Could you check a few things on this model? Use its own coordinates, in mm. Give positions to 0.01 mm unless a question says otherwise; leave off trailing zeros. Order: outer loops, then holes, each group sorted by start corner. A loop starts at its lowest first (then second) coordinate and runs counter-clockwise, first axis right, second up. Notation, with made-up numbers: M 72,18 L 94,18 A12 ccw 94,39 Z; hole C 10,65.5 d4. An arc over 180 degrees is marked long. Answer in a Markdown table with one row per item. Add a question column.
```python
from build123d import *

# Parameters (mm, degrees)
SKETCH1_W           = 203.2
SKETCH1_H           = 133.35
BOSS_EXTRUDE1_DEPTH = 3.175
SKETCH2_R           = 2.54
CUT_EXTRUDE1_DEPTH  = 122.565604716
SKETCH3_W           = 35.687
SKETCH3_H           = 3.175
BOSS_EXTRUDE2_DEPTH = 3.175
SKETCH4_W           = 3.175
SKETCH4_H           = 18.542
BOSS_EXTRUDE3_DEPTH = 3.175
BOSS_EXTRUDE4_DEPTH = 3.175
SKETCH6_W           = 76.708
SKETCH6_H           = 51.308
CUT_EXTRUDE2_DEPTH  = 126.963898598


with BuildPart() as part:
    # Sketch1 → Boss-Extrude1 (new body)
    with BuildSketch(Plane(origin=(0, 0, 0), x_dir=(1, 0, 0), z_dir=(0, 1, 0))):
        Rectangle(SKETCH1_W, SKETCH1_H)
    extrude(amount=BOSS_EXTRUDE1_DEPTH)

    # Sketch2 → Cut-Extrude1 (cut, through all)
    with BuildSketch(Plane(origin=(0, 3.175, 0), x_dir=(1, 0, 0), z_dir=(0, 1, 0))):
        with Locations(Location((-88.9, 50.8, 0), (0, 0, 270))):
            Circle(SKETCH2_R)
        with Locations(Location((-76.2, 50.8, 0), (0, 0, 270))):
            Circle(SKETCH2_R)
        with Locations(Location((-63.5, 50.8, 0), (0, 0, 270))):
            Circle(SKETCH2_R)
        with Locations(Location((-50.8, 50.8, 0), (0, 0, 270))):
            Circle(SKETCH2_R)
        with Locations(Location((-76.2, 38.1, 0), (0, 0, 270))):
            Circle(SKETCH2_R)
        with Locations(Location((-63.5, 38.1, 0), (0, 0, 270))):
            Circle(SKETCH2_R)
        with Locations(Location((-50.8, 38.1, 0), (0, 0, 270))):
            Circle(SKETCH2_R)
        with Locations(Location((-76.2, 25.4, 0), (0, 0, 270))):
            Circle(SKETCH2_R)
        with Locations(Location((-63.5, 25.4, 0), (0, 0, 270))):
            Circle(SKETCH2_R)
        with Locations(Location((-50.8, 25.4, 0), (0, 0, 270))):
            Circle(SKETCH2_R)
        with Locations(Location((-76.2, 12.7, 0), (0, 0, 270))):
            Circle(SKETCH2_R)
        with Locations(Location((-63.5, 12.7, 0), (0, 0, 270))):
            Circle(SKETCH2_R)
        with Locations(Location((-50.8, 12.7, 0), (0, 0, 270))):
            Circle(SKETCH2_R)
        with Locations(Location((-76.2, 0, 0), (0, 0, 270))):
            Circle(SKETCH2_R)
        with Locations(Location((-63.5, 0, 0), (0, 0, 270))):
            Circle(SKETCH2_R)
        with Locations(Location((-50.8, 0, 0), (0, 0, 270))):
            Circle(SKETCH2_R)
        with Locations(Location((-76.2, -12.7, 0), (0, 0, 270))):
            Circle(SKETCH2_R)
        with Locations(Location((-63.5, -12.7, 0), (0, 0, 270))):
            Circle(SKETCH2_R)
        with Locations(Location((-50.8, -12.7, 0), (0, 0, 270))):
            Circle(SKETCH2_R)
        with Locations(Location((-76.2, -25.4, 0), (0, 0, 270))):
            Circle(SKETCH2_R)
        with Locations(Location((-63.5, -25.4, 0), (0, 0, 270))):
            Circle(SKETCH2_R)
        with Locations(Location((-50.8, -25.4, 0), (0, 0, 270))):
            Circle(SKETCH2_R)
        with Locations(Location((-76.2, -38.1, 0), (0, 0, 270))):
            Circle(SKETCH2_R)
        with Locations(Location((-63.5, -38.1, 0), (0, 0, 270))):
            Circle(SKETCH2_R)
        with Locations(Location((-50.8, -38.1, 0), (0, 0, 270))):
            Circle(SKETCH2_R)
        with Locations(Location((-76.2, -50.8, 0), (0, 0, 270))):
            Circle(SKETCH2_R)
        with Locations(Location((-63.5, -50.8, 0), (0, 0, 270))):
            Circle(SKETCH2_R)
        with Locations(Location((-50.8, -50.8, 0), (0, 0, 270))):
            Circle(SKETCH2_R)
        with Locations(Location((-88.9, 38.1, 0), (0, 0, 270))):
            Circle(SKETCH2_R)
        with Locations(Location((-88.9, 25.4, 0), (0, 0, 270))):
            Circle(SKETCH2_R)
        with Locations(Location((-88.9, 12.7, 0), (0, 0, 270))):
            Circle(SKETCH2_R)
        with Locations(Location((-88.9, 0, 0), (0, 0, 270))):
            Circle(SKETCH2_R)
        with Locations(Location((-88.9, -12.7, 0), (0, 0, 270))):
            Circle(SKETCH2_R)
        with Locations(Location((-88.9, -25.4, 0), (0, 0, 270))):
            Circle(SKETCH2_R)
        with Locations(Location((-88.9, -38.1, 0), (0, 0, 270))):
            Circle(SKETCH2_R)
        with Locations(Location((-88.9, -50.8, 0), (0, 0, 270))):
            Circle(SKETCH2_R)
        with Locations(Location((-38.1, 50.8, 0), (0, 0, 270))):
            Circle(SKETCH2_R)
        with Locations(Location((-38.1, 38.1, 0), (0, 0, 270))):
            Circle(SKETCH2_R)
        with Locations(Location((-38.1, 25.4, 0), (0, 0, 270))):
            Circle(SKETCH2_R)
        with Locations(Location((-38.1, 12.7, 0), (0, 0, 270))):
            Circle(SKETCH2_R)
        with Locations(Location((-38.1, 0, 0), (0, 0, 270))):
            Circle(SKETCH2_R)
        with Locations(Location((-38.1, -12.7, 0), (0, 0, 270))):
            Circle(SKETCH2_R)
        with Locations(Location((-38.1, -25.4, 0), (0, 0, 270))):
            Circle(SKETCH2_R)
        with Locations(Location((-38.1, -38.1, 0), (0, 0, 270))):
            Circle(SKETCH2_R)
        with Locations(Location((-38.1, -50.8, 0), (0, 0, 270))):
            Circle(SKETCH2_R)
    extrude(amount=-CUT_EXTRUDE1_DEPTH, mode=Mode.SUBTRACT)

    # Sketch3 → Boss-Extrude2 (add)
    with BuildSketch(Plane(origin=(0, 3.175, 0), x_dir=(1, 0, 0), z_dir=(0, 1, 0))):
        with Locations((-61.2775, 68.2625)):
            Rectangle(SKETCH3_W, SKETCH3_H)
        with Locations((0.3175, 68.2625)):
            Rectangle(SKETCH3_W, SKETCH3_H)
        with Locations((61.9125, 68.2625)):
            Rectangle(SKETCH3_W, SKETCH3_H)
        with Locations((61.9125, -68.2625)):
            Rectangle(SKETCH3_W, SKETCH3_H)
        with Locations((0.3175, -68.2625)):
            Rectangle(SKETCH3_W, SKETCH3_H)
        with Locations((-61.2775, -68.2625)):
            Rectangle(SKETCH3_W, SKETCH3_H)
    extrude(amount=-BOSS_EXTRUDE2_DEPTH)

    # Sketch4 → Boss-Extrude3 (add)
    with BuildSketch(Plane(origin=(0, 3.175, 0), x_dir=(1, 0, 0), z_dir=(0, 1, 0))):
        with Locations((-103.1875, 38.1)):
            Rectangle(SKETCH4_W, SKETCH4_H)
        with Locations((-103.1875, 0)):
            Rectangle(SKETCH4_W, SKETCH4_H)
        with Locations((-103.1875, -38.1)):
            Rectangle(SKETCH4_W, SKETCH4_H)
        with Locations((103.1875, -38.1)):
            Rectangle(SKETCH4_W, SKETCH4_H)
        with Locations((103.1875, 0)):
            Rectangle(SKETCH4_W, SKETCH4_H)
        with Locations((103.1875, 38.1)):
            Rectangle(SKETCH4_W, SKETCH4_H)
    extrude(amount=-BOSS_EXTRUDE3_DEPTH)

    # Sketch5 → Boss-Extrude4 (add)
    with BuildSketch(Plane(origin=(0, 3.175, 0), x_dir=(1, 0, 0), z_dir=(0, 1, 0))):
        Polygon((-104.775, -47.371), (-104.775, -69.85), (-79.121, -69.85), (-79.121, -66.675), (-101.6, -66.675), (-101.6, -47.371), align=None)
        Polygon((-101.6, 47.371), (-104.775, 47.371), (-104.775, 69.85), (-79.121, 69.85), (-79.121, 66.675), (-101.6, 66.675), align=None)
        Polygon((104.775, 47.371), (104.775, 69.85), (79.121, 69.85), (79.121, 66.675), (101.6, 66.675), (101.6, 47.371), align=None)
        Polygon((101.6, -47.371), (104.775, -47.371), (104.775, -69.85), (79.121, -69.85), (79.121, -66.675), (101.6, -66.675), align=None)
    extrude(amount=-BOSS_EXTRUDE4_DEPTH)

    # Sketch6 → Cut-Extrude2 (cut, through all)
    with BuildSketch(Plane(origin=(0, 3.175, 0), x_dir=(1, 0, 0), z_dir=(0, 1, 0))):
        with Locations((25.4, 0)):
            Rectangle(SKETCH6_W, SKETCH6_H)
    extrude(amount=-CUT_EXTRUDE2_DEPTH, mode=Mode.SUBTRACT)


solid = part.part
```
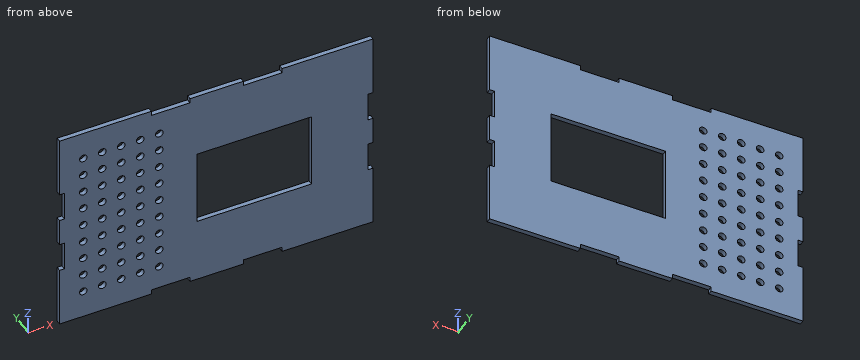
1. If I drill on line 1 along X through (y, z) = (1.45, -50.8) (3 decimals); line 2 along X through (y, z) = (2.65, -37) (3 decimals); line 3 along X through (y, z) = (1.25, 18.5), over which ranges is the centre line in solid material (lowest first)? Write a range as [from, to].
2. Suppose I cut it at B-B on x = 39.5. List the corners of the cut face in (y, z) for me (3 decimals).
3. Suppose I cut it at D-D on y = 1.5. Count the separate pieces of the cut face and the enclosed holes in it, plus the area to 3 significant figures.
4. Will this pin go through, and if not, where does the flat tip stop? P1, Ø1, axis at x = -29.5, y = 1.5, coming from the -Z side (3 decimals).
5. Suppose I cut it at C-C on z = -50.8. List the corners of the cut face in (x, y) for me (3 decimals).
6. Suppose I cut it at A-A on z = -12.7. List the corners of the cut face in (x, y) for me (3 decimals).
Findings below:
| question | item | result |
|---|---|---|
| 1 | line 1 | [-104.775, -91.44], [-86.36, -78.74], [-73.66, -66.04], [-60.96, -53.34], [-48.26, -40.64], [-35.56, 104.775] |
| 1 | line 2 | [-104.775, -91.189], [-86.611, -78.489], [-73.911, -65.789], [-61.211, -53.089], [-48.511, -40.389], [-35.811, 104.775] |
| 1 | line 3 | [-101.6, -12.95], [63.75, 101.6] |
| 2 | outline | M 0,-66.675 L 3.175,-66.675 L 3.175,-25.654 L 0,-25.654 Z; M 0,25.654 L 3.175,25.654 L 3.175,66.675 L 0,66.675 Z |
| 3 | separate pieces | 1 |
| 3 | enclosed holes | 46 |
| 3 | area | 23,800 mm2 |
| 4 | P1 | z = -66.675 |
| 5 | outline | M -104.775,0 L -91.44,0 L -91.44,3.175 L -104.775,3.175 Z; M -86.36,0 L -78.74,0 L -78.74,3.175 L -86.36,3.175 Z; M -73.66,0 L -66.04,0 L -66.04,3.175 L -73.66,3.175 Z; M -60.96,0 L -53.34,0 L -53.34,3.175 L -60.96,3.175 Z; M -48.26,0 L -40.64,0 L -40.64,3.175 L -48.26,3.175 Z; M -35.56,0 L 104.775,0 L 104.775,3.175 L -35.56,3.175 Z |
| 6 | outline | M -101.6,0 L -91.44,0 L -91.44,3.175 L -101.6,3.175 Z; M -86.36,0 L -78.74,0 L -78.74,3.175 L -86.36,3.175 Z; M -73.66,0 L -66.04,0 L -66.04,3.175 L -73.66,3.175 Z; M -60.96,0 L -53.34,0 L -53.34,3.175 L -60.96,3.175 Z; M -48.26,0 L -40.64,0 L -40.64,3.175 L -48.26,3.175 Z; M -35.56,0 L -12.954,0 L -12.954,3.175 L -35.56,3.175 Z; M 63.754,0 L 101.6,0 L 101.6,3.175 L 63.754,3.175 Z |
